Drawing for the job (mm, zero at the part's lowest x, y, z). A direction names the side the tool comes from. Round coordinates to 2 decimals unless told otherwise and drop trailing zeros. Loops run counter-clockwise (first coordinate to the right, second up) from the corner with the lowest first, then second, coordinate; pieces in that order, holes last. Notation, with made-up numbers: M 38,49 L 64,49 A21 ccw 64,75 Z; hole C 43,11.25 d2. An arc over 180 degrees is marked long. Write each question's results on one line, items separated by ' | '.
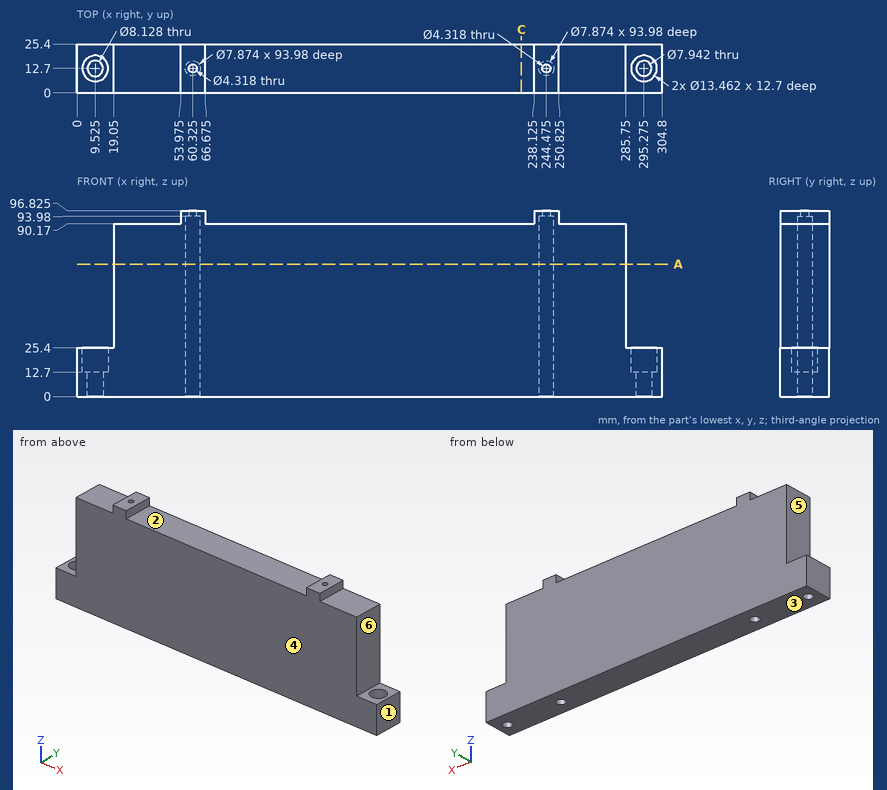
Item 1: Drop flat-ended pins along their axis: P1, Ø7.5, axis at y = 15, z = 94, coming from the -X side (3 decimals); P2, Ø5, axis at x = 98.5, y = 15.5, coming from the +Z side; P3, Ø2, axis at y = 6.5, z = 80, coming from the +X side; P4, Ø2, axis at x = 146.5, z = 24.5, coming from the -Y side. Give the stop position or say it passes through.
Filled sheet:
P1: x = 53.975 | P2: z = 90.17 | P3: x = 285.75 | P4: y = 0
Item 2: Which spindle directions (+Z, -Z, +X, -X, +Y, -Y) get a long thin tool onto all of the face, cutting with end or side? Do the marked faces 4, 5 and 6. Say none if no direction does.
Filled sheet:
face 4: +Z, -Z, +X, -X, -Y | face 5: +Z, -X, +Y, -Y | face 6: +Z, +X, +Y, -Y
Item 3: Two-plate mould, pull along X, no slides. Class the marked faces 1, 2 and 3: +X half, -X half, draft (parallel to the pull), parting line (faces both ways), or undercut.
Filled sheet:
face 1: +X half | face 2: undercut | face 3: draft
Item 4: Band-saw the part on A-A on z = 69. Count the separate pieces of the cut face and the enclosed holes in it, and give its area (3 significant figures).
Filled sheet:
separate pieces: 1 | enclosed holes: 2 | area: 6,680 mm^2
Item 5: Wall check: L1, parallel to X at y = 12, z = 57.5; L2, parallel to X at y = 12.7, z = 95.65 (1 decimal); L3, parallel to X at y = 12.7, z = 40. Give the ranges that are in metal, low to high.
Filled sheet:
L1: 19.05 to 56.45, 64.2 to 240.6, 248.35 to 285.75 | L2: 54 to 58.2, 62.5 to 66.7, 238.1 to 242.3, 246.6 to 250.8 | L3: 19.05 to 56.39, 64.26 to 240.54, 248.41 to 285.75
Item 6: Band-saw the part on C-C on x = 231.5. Give the cut face in (y, z), and give its area (3 significant figures).
Filled sheet:
outline: M 0,0 L 25.4,0 L 25.4,90.17 L 0,90.17 Z | area: 2,290 mm^2
